Here's how the part is built. I have some questions about the finished solid (model axes, mm). Face numbers are marked on the shaded views. A direction names the side the tool comes from. Round coordinates to 2 decimals unless told otherwise and drop trailing zeros. Write each loop counter-clockwise with the first axis right and the second up, starting at its lowest first coordinate (ties: lowest second). Pieces come first, ordered by that corner, then holes. Notation, with made-up numbers: (29.5, 62.5) - (63.5, 62.5) arc R22 cw to (63.5, 83.5) - close; hole circle Ø7 at (-3.75, 67). An arc over 180 degrees is marked (long way). Write item = value, one per line. Start each with the question number.
Item 1: For P1, Ø4, axis at x = -26, z = 9, coming from the -Y side; P2, Ø3, axis at x = -13, y = -16, coming from the -Z side, each with a flat end and sliding along its axis, tell me the tip position at first contact or that it passes through.
Item 2: Which directions (+Z, -Z, +X, -X, +Y, -Y) give clear straight access to the entire face, cutting with the end or side of a thin tool? Please do the marked faces 5 and 6.
Item 3: If we section it at A-A (z = 1.25): Please give me the cut outline in (x, y).
Item 4: If we section it at B-B (x = -12.25): Please give me the cut outline in (y, z).
Item 5: If I drill on line 1 along X through (y, z) = (-18, 2.25); line 2 along X through (y, z) = (8, 7.75); line 3 along X through (y, z) = (8.5, 3.25), over which ranges is the centre line in solid material (lowest first)? Write a range as [from, to].
Item 6: If we section it at D-D (z = 5.75): Please give me the cut outline in (x, y).
Item 7: Thinking about a two-plate mould opening in X: for the marked faces 1, 2, 3 and 4, which applies, pulls with the +X half, pulls with the -X half, needs draft (parallel to the pull), parting line crosses it, or undercut?
Item 8: If we section it at C-C (x = -22.25): Please give me the cut outline in (y, z).
```python
from build123d import *

# Parameters (mm, degrees)
ESQUISSE1_W             = 21
ESQUISSE1_H             = 45
BOSS_EXTRU_1_DEPTH      = 10
ESQUISSE2_R             = 2.5
ENL_V_MAT_EXTRU_1_DEPTH = 10
ESQUISSE4_R             = 2
ENL_V_MAT_EXTRU_3_DEPTH = 10
CONG_1_R                = 5
ENL_V_MAT_EXTRU_6_DEPTH = 4


with BuildPart() as part:
    # Esquisse1 → Boss.-Extru.1 (new body)
    with BuildSketch(Plane.XY):
        with Locations((-17.606794518, -4.650313152)):
            Rectangle(ESQUISSE1_W, ESQUISSE1_H)
    extrude(amount=BOSS_EXTRU_1_DEPTH)

    # Esquisse2 → Enlèv. mat.-Extru.1 (cut)
    with BuildSketch(Plane.XY.offset(10)):
        with Locations((-23.106794518, 7.849686848)):
            Circle(ESQUISSE2_R)
    extrude(amount=-ENL_V_MAT_EXTRU_1_DEPTH, mode=Mode.SUBTRACT)

    # Esquisse4 → Enlèv. mat.-Extru.3 (cut)
    with BuildSketch(Plane.XY.offset(10)):
        with Locations((-13.106794518, 7.849686848)):
            Circle(ESQUISSE4_R)
        with Locations((-13.106794518, -17.150313152)):
            Circle(ESQUISSE4_R)
    extrude(amount=-ENL_V_MAT_EXTRU_3_DEPTH, mode=Mode.SUBTRACT)

    # Congé1
    cong_1_edges = [part.edges().sort_by_distance(p)[0] for p in [
        (-28.106794518, 17.849686848, 5),
        (-28.106794518, -27.150313152, 5),
    ]]
    fillet(cong_1_edges, radius=CONG_1_R)

    # Esquisse7 → Enlèv. mat.-Extru.6 (cut)
    with BuildSketch(Plane(origin=(0, 0, 0), x_dir=(-1, 0, 0), z_dir=(0, 0, -1))):
        Polygon((15.856794518, 9.437400088), (13.106794518, 11.025113328), (10.356794518, 9.437400088), (10.356794518, 6.261973607), (13.106794518, 4.674260367), (15.856794518, 6.261973607), align=None)
        Polygon((15.856794518, -15.562599912), (13.106794518, -13.974886672), (10.356794518, -15.562599912), (10.356794518, -18.738026393), (13.106794518, -20.325739633), (15.856794518, -18.738026393), align=None)
    extrude(amount=-ENL_V_MAT_EXTRU_6_DEPTH, mode=Mode.SUBTRACT)


solid = part.part
```
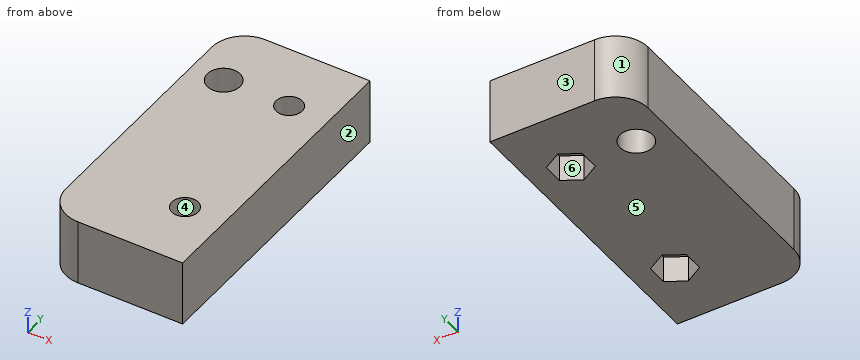
Reply:
q1.P1 = -27.07
q1.P2 = 4
q2.face_5 = -Z, +X, -X, +Y, -Y
q2.face_6 = -Z
q3.outline = (-28.11, -22.15) arc R5 ccw to (-23.11, -27.15) - (-7.11, -27.15) - (-7.11, 17.85) - (-23.11, 17.85) arc R5 ccw to (-28.11, 12.85) - close; hole circle Ø5 at (-23.11, 7.85); hole (-15.86, -18.74) - (-13.11, -20.33) - (-10.36, -18.74) - (-10.36, -15.56) - (-13.11, -13.97) - (-15.86, -15.56) - close; hole (-15.86, 6.26) - (-13.11, 4.67) - (-10.36, 6.26) - (-10.36, 9.44) - (-13.11, 11.03) - (-15.86, 9.44) - close
q4.outline = (-27.15, 0) - (-19.83, 0) - (-19.83, 4) - (-18.96, 4) - (-18.96, 10) - (-27.15, 10) - close; (-15.34, 4) - (-14.47, 4) - (-14.47, 0) - (5.17, 0) - (5.17, 4) - (6.04, 4) - (6.04, 10) - (-15.34, 10) - close; (9.66, 4) - (10.53, 4) - (10.53, 0) - (17.85, 0) - (17.85, 10) - (9.66, 10) - close
q5.line_1 = [-28.11, -15.86], [-10.36, -7.11]
q5.line_2 = [-28.11, -25.6], [-20.61, -15.1], [-11.11, -7.11]
q5.line_3 = [-28.11, -25.52], [-20.69, -15.86], [-10.36, -7.11]
q6.outline = (-28.11, -22.15) arc R5 ccw to (-23.11, -27.15) - (-7.11, -27.15) - (-7.11, 17.85) - (-23.11, 17.85) arc R5 ccw to (-28.11, 12.85) - close; hole circle Ø5 at (-23.11, 7.85); hole circle Ø4 at (-13.11, -17.15); hole circle Ø4 at (-13.11, 7.85)
q7.face_1 = pulls with the -X half
q7.face_2 = pulls with the +X half
q7.face_3 = needs draft
q7.face_4 = undercut
q8.outline = (-27.15, 0) - (5.5, 0) - (5.5, 10) - (-27.15, 10) - close; (10.2, 0) - (17.85, 0) - (17.85, 10) - (10.2, 10) - close
